Design review of the part built by this model. Coordinates are the model's own, in mm. Face numbers are marked on the shaded views. A direction names the side the tool comes from. Coordinates: 2 decimals unless noted, no trailing zeros. Loops run counter-clockwise (first coordinate to the right, second up) from the corner with the lowest first, then second, coordinate; pieces in that order, holes last. Notation, with made-up numbers: (-24.5, -10.5) -> (-4.5, -10.5) arc R19 cw to (-4.5, 20.5) -> close; hole circle Ø4 at (14, 31.25). An arc over 180 degrees is marked (long way). Answer in a Markdown table with one row per item.
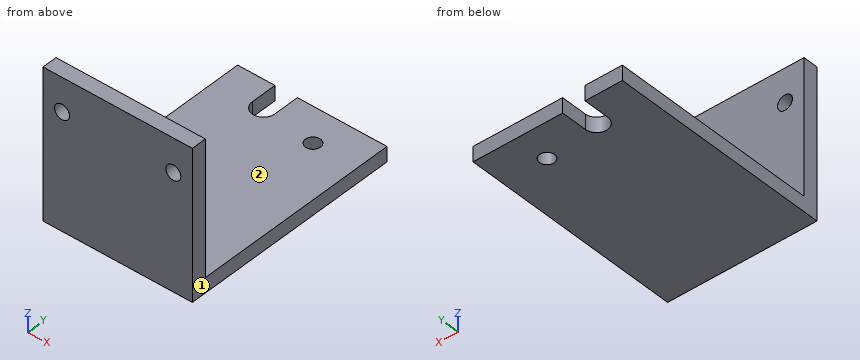
```python
from build123d import *

# Parameters (mm, degrees)
CYLINDER002_R     = 2
CYLINDER002_DEPTH = 4
CYLINDER003_R     = 3
CYLINDER003_DEPTH = 4
BOX002_W          = 6
BOX002_H          = 7
BOX002_DEPTH      = 4
CYLINDER_R        = 2
CYLINDER_DEPTH    = 4
CYLINDER001_R     = 2
CYLINDER001_DEPTH = 4
BOX_W             = 40
BOX_H             = 60
BOX_DEPTH         = 4
BOX001_W          = 40
BOX001_H          = 4
BOX001_DEPTH      = 40


with BuildPart() as obj1:
    # Cylinder002 → Cylinder002 (new body)
    with BuildSketch(Plane(origin=(28, 51, 0), x_dir=(1, 0, 0), z_dir=(0, 0, 1))):
        Circle(CYLINDER002_R)
    extrude(amount=CYLINDER002_DEPTH)


with BuildPart() as cilindro003:
    # Cylinder003 → Cylinder003 (new body)
    with BuildSketch(Plane(origin=(13, 53, 0), x_dir=(1, 0, 0), z_dir=(0, 0, 1))):
        Circle(CYLINDER003_R)
    extrude(amount=CYLINDER003_DEPTH)


with BuildPart() as obj1_del_hotend:
    # Box002 → Box002 (new body)
    with BuildSketch(Plane(origin=(10, 53, 0), x_dir=(1, 0, 0), z_dir=(0, 0, 1))):
        with Locations((3, 3.5)):
            Rectangle(BOX002_W, BOX002_H)
    extrude(amount=BOX002_DEPTH)

    # Fusion002: union Cilindro003
    add(cilindro003.part)


with BuildPart() as cylinder:
    # Cylinder → Cylinder (new body)
    with BuildSketch(Plane(origin=(5.1, 4, 31), x_dir=(0, 0, 1), z_dir=(0, -1, 0))):
        Circle(CYLINDER_R)
    extrude(amount=CYLINDER_DEPTH)


with BuildPart() as agujeros_roscados_m4:
    # Cylinder001 → Cylinder001 (new body)
    with BuildSketch(Plane(origin=(34.9, 4, 31), x_dir=(0, 0, 1), z_dir=(0, -1, 0))):
        Circle(CYLINDER001_R)
    extrude(amount=CYLINDER001_DEPTH)

    # Fusion001: union Cylinder
    add(cylinder.part)


with BuildPart() as cubo:
    # Box → Box (new body)
    with BuildSketch(Plane.XY):
        with Locations((20, 30)):
            Rectangle(BOX_W, BOX_H)
    extrude(amount=BOX_DEPTH)


with BuildPart() as obj2:
    # Box001 → Box001 (new body)
    with BuildSketch(Plane.XY):
        with Locations((20, 2)):
            Rectangle(BOX001_W, BOX001_H)
    extrude(amount=BOX001_DEPTH)

    # Fusion: union Cubo
    add(cubo.part)

    # Cut: cut Agujeros roscados M4
    add(agujeros_roscados_m4.part, mode=Mode.SUBTRACT)

    # Cut001: cut obj1_del_hotend
    add(obj1_del_hotend.part, mode=Mode.SUBTRACT)

    # Cut002: cut obj1
    add(obj1.part, mode=Mode.SUBTRACT)


solid = obj2.part
```
(1) Take a section at B-B on z = 31. Give the boundary of the cut face in (x, y), and give its area (3 significant figures).
Evaluation:
| item | result |
|---|---|
| outline | (0, 0) -> (3.1, 0) -> (3.1, 4) -> (0, 4) -> close; (7.1, 0) -> (32.9, 0) -> (32.9, 4) -> (7.1, 4) -> close; (36.9, 0) -> (40, 0) -> (40, 4) -> (36.9, 4) -> close |
| area | 128 mm² |
(2) Tool access review of the marked faces 1 and 2: name each direction out of +Z, -Z, +X, -X, +Y, -Y from which nothing blocks a thin tool from reaching the whole face with its end or side.
Evaluation:
| item | result |
|---|---|
| face 1 | +Z, -Z, +X, +Y, -Y |
| face 2 | +Z, +X, -X, +Y |
(3) Take a section at A-A on x = 34.9. Give the boundary of the cut face in (y, z).
Evaluation:
| item | result |
|---|---|
| outline | (0, 0) -> (60, 0) -> (60, 4) -> (4, 4) -> (4, 29) -> (0, 29) -> close; (0, 33) -> (4, 33) -> (4, 40) -> (0, 40) -> close |
(4) Take a section at D-D on x = 29. Give the boundary of the cut face in (y, z).
Evaluation:
| item | result |
|---|---|
| outline | (0, 0) -> (49.27, 0) -> (49.27, 4) -> (4, 4) -> (4, 40) -> (0, 40) -> close; (52.73, 0) -> (60, 0) -> (60, 4) -> (52.73, 4) -> close |
(5) Take a section at C-C on y = 51. Give the boundary of the cut face in (x, z).
Evaluation:
| item | result |
|---|---|
| outline | (0, 0) -> (10.76, 0) -> (10.76, 4) -> (0, 4) -> close; (15.24, 0) -> (26, 0) -> (26, 4) -> (15.24, 4) -> close; (30, 0) -> (40, 0) -> (40, 4) -> (30, 4) -> close |
(6) To check wall thickness, follow probe 1 along X at (y, z) = (1.1, 31); probe 2 along Z at (x, y) = (5.1, 3.2); probe 3 along Y at (x, z) = (28, 2). State the ranges of each line that lie inside material, in increasing order.
Evaluation:
| item | result |
|---|---|
| probe 1 | x = 0 to 3.1, 7.1 to 32.9, 36.9 to 40 |
| probe 2 | z = 0 to 29, 33 to 40 |
| probe 3 | y = 0 to 49, 53 to 60 |
(7) For pin 1 (10 mm diameter, centred on x = 10.5, z = 19, fed in from -Y); pin 2 (1.5 mm diameter, centred on x = 13, z = 10.5, fed in from +Y); pin 3 (2 mm diameter, centred on x = 20.5, y = 49.5, fed in from +Z), all flat-tipped, find the tip position at first contact; note any pin that passes through.
Evaluation:
| item | result |
|---|---|
| pin 1 | stops at y = 0 |
| pin 2 | stops at y = 4 |
| pin 3 | stops at z = 4 |
